Build history of the part. All positions in model axes, mm. Round coordinates to 2 decimals unless told otherwise and drop trailing zeros. Write each loop counter-clockwise with the first axis right and the second up, starting at its lowest first coordinate (ties: lowest second). Pieces come first, ordered by that corner, then holes.
from build123d import *

# Parameters (mm, degrees)
SKETCH_1_R          = 14.5
EXTRUDE_1_DEPTH     = 6
SKETCH_2_R          = 2.5
CUT_EXTRUDE_1_DEPTH = 10
FILLET_1_R          = 7
FILLET_2_R          = 7


with BuildPart() as part:
    # Эскиз1 → Бобышка-Вытянуть1 (new body)
    with BuildSketch(Plane(origin=(0, 0, 0), x_dir=(1, 0, 0), z_dir=(0, 1, 0))):
        with BuildLine():
            Line((60.2245797, -27), (46.823097933, -27))
            ThreePointArc((46.823097933, -27), (-54.05, 0), (46.823097933, 27))
            Line((46.823097933, 27), (60.2245797, 27))
            ThreePointArc((60.2245797, 27), (66, 0), (60.2245797, -27))
        make_face()
        with Locations(Location((0, 0, 0), (0, 0, 270))):
            Circle(SKETCH_1_R, mode=Mode.SUBTRACT)
    extrude(amount=EXTRUDE_1_DEPTH)

    # Эскиз2 → Вырез-Вытянуть1 (cut)
    with BuildSketch(Plane(origin=(0, 6, 0), x_dir=(1, 0, 0), z_dir=(0, 1, 0))):
        with Locations(Location((0, 42.5, 0), (0, 0, 270))):
            Circle(SKETCH_2_R)
        with Locations(Location((0, -42.5, 0), (0, 0, 270))):
            Circle(SKETCH_2_R)
        with Locations(Location((-42.5, 0, 0), (0, 0, 270))):
            Circle(SKETCH_2_R)
        with Locations(Location((42.5, 0, 0), (0, 0, 270))):
            Circle(SKETCH_2_R)
    extrude(amount=-CUT_EXTRUDE_1_DEPTH, mode=Mode.SUBTRACT)

    # Скругление1
    fillet_1_edges = [part.edges().sort_by_distance(p)[0] for p in [
        (60.2245797, 3, -27),
        (60.2245797, 3, 27),
    ]]
    fillet(fillet_1_edges, radius=FILLET_1_R)

    # Скругление2
    fillet_2_edges = [part.edges().sort_by_distance(p)[0] for p in [
        (46.823097933, 3, -27),
        (46.823097933, 3, 27),
    ]]
    fillet(fillet_2_edges, radius=FILLET_2_R)


solid = part.part
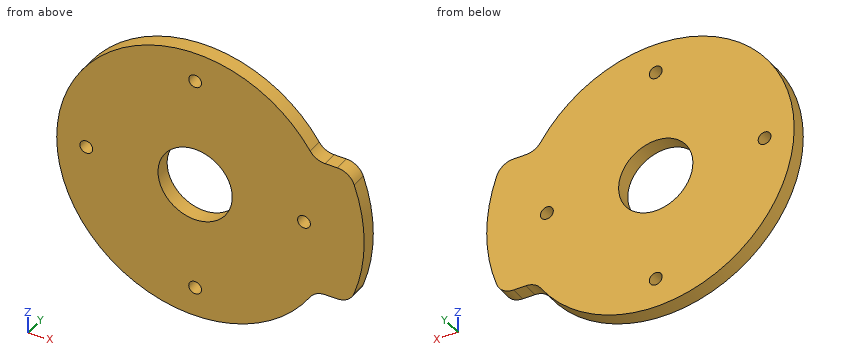
1) Wall check: L1, parallel to X at y = 3.8, z = 0; L2, parallel to X at y = 0.5, z = 1; L3, parallel to Z at x = 2, y = 3.3. Give the ranges that are in metal, low to high.
Results:
L1: x = -54.05 to -45, -40 to -14.5, 14.5 to 40, 45 to 66
L2: x = -54.04 to -44.79, -40.21 to -14.47, 14.47 to 40.21, 44.79 to 65.99
L3: z = -54.01 to -44, -41 to -14.36, 14.36 to 41, 44 to 54.01
2) Slice it at A-A (x = 0). Write the cut outline in (y, z), plus the area to 3 significant figures.
Results:
outline: (0, -54.05) - (6, -54.05) - (6, -45) - (0, -45) - close; (0, -40) - (6, -40) - (6, -14.5) - (0, -14.5) - close; (0, 14.5) - (6, 14.5) - (6, 40) - (0, 40) - close; (0, 45) - (6, 45) - (6, 54.05) - (0, 54.05) - close
area: 415 mm2
3) Slice it at B-B (z = 0). Write the cut outline in (x, y).
Results:
outline: (-54.05, 0) - (-45, 0) - (-45, 6) - (-54.05, 6) - close; (-40, 0) - (-14.5, 0) - (-14.5, 6) - (-40, 6) - close; (14.5, 0) - (40, 0) - (40, 6) - (14.5, 6) - close; (45, 0) - (66, 0) - (66, 6) - (45, 6) - close
4) Pin check, flat tips, straight feed: pin 1 Ø1 at (x, y) = (-27.5, 2.5) entering from -Z; pin 2 Ø3 at (y, z) = (4.5, 36.5) entering from +X; pin 3 Ø3 at (x, z) = (0, 42.5) entering from +Y; pin 4 Ø2.5 at (x, y) = (54, 4.5) entering from +Z. Stop position of each tip, or through.
Results:
pin 1: stops at z = -46.82
pin 2: stops at x = 41.19
pin 3: passes through
pin 4: stops at z = 27
5) Slice it at C-C (y = 4). Write the cut outline in (x, z).
Results:
outline: (44.89, -30.1) arc R7 cw to (50.71, -27) - (55.51, -27) arc R7 ccw to (62.09, -22.37) arc R66 ccw to (62.09, 22.37) arc R7 ccw to (55.51, 27) - (50.71, 27) arc R7 cw to (44.89, 30.1) arc R54.05 ccw (long way) to start; hole circle Ø5 at (-42.5, 0); hole circle Ø29 at (0, 0); hole circle Ø5 at (0, -42.5); hole circle Ø5 at (0, 42.5); hole circle Ø5 at (42.5, 0)
6) Slice it at D-D (z = -11.5). Write the cut outline in (x, y).
Results:
outline: (-52.81, 0) - (-8.83, 0) - (-8.83, 6) - (-52.81, 6) - close; (8.83, 0) - (64.99, 0) - (64.99, 6) - (8.83, 6) - close
